from build123d import *

# Parameters (mm, degrees)
EXTRUDE_2_DEPTH     = 60
CUT_EXTRUDE_2_DEPTH = 189.939286944
SKETCH_7_R          = 25
CUT_EXTRUDE_4_DEPTH = 20
SKETCH_8_R          = 25
CUT_EXTRUDE_5_DEPTH = 20
SKETCH_9_W          = 30
SKETCH_9_H          = 70
CUT_EXTRUDE_6_DEPTH = 20
SKETCH_10_W         = 30
SKETCH_10_H         = 70
CUT_EXTRUDE_7_DEPTH = 20
FILLET_1_R          = 3
FILLET_2_R          = 3
FILLET_3_R          = 3
FILLET_4_R          = 3


with BuildPart() as part:
    # 草图1 → 凸台-拉伸2 (new body)
    with BuildSketch(Plane.XY):
        Polygon((-161.784091828, 76.967277349), (-161.784091828, 16.967277349), (-127.826106531, -63.032722651), (-27.826106531, -63.032722651), (6.131878766, 16.967277349), (6.131878766, 76.967277349), align=None)
    extrude(amount=EXTRUDE_2_DEPTH)

    # 草图5 → 切除-拉伸2 (cut, through all)
    with BuildSketch(Plane.XY.offset(60)):
        Polygon((-141.784091828, 76.967277349), (-141.784091828, 16.967277349), (-112.836441026, -51.229114277), (-42.815772036, -51.229114277), (-13.868121234, 16.967277349), (-13.868121234, 76.967277349), align=None)
    extrude(amount=-CUT_EXTRUDE_2_DEPTH, mode=Mode.SUBTRACT)

    # 草图7 → 切除-拉伸4 (cut)
    with BuildSketch(Plane.ZY.offset(161.784091828)):
        with Locations(Location((30, 46.967277349, 0), (0, 0, 270))):
            Circle(SKETCH_7_R)
    extrude(amount=-CUT_EXTRUDE_4_DEPTH, mode=Mode.SUBTRACT)

    # 草图8 → 切除-拉伸5 (cut)
    with BuildSketch(Plane(origin=(0, -51.229114277, 0), x_dir=(1, 0, 0), z_dir=(0, 1, 0))):
        with Locations(Location((-77.815772036, -30, 0), (0, 0, 270))):
            Circle(SKETCH_8_R)
    extrude(amount=-CUT_EXTRUDE_5_DEPTH, mode=Mode.SUBTRACT)

    # 草图9 → 切除-拉伸6 (cut)
    with BuildSketch(Plane(origin=(-130.981763761, -55.598460099, 0), x_dir=(0, 0, 1), z_dir=(-0.9205048534524416, -0.3907311284892711, 0))):
        with Locations((30, 36.923711729)):
            Rectangle(SKETCH_9_W, SKETCH_9_H)
    extrude(amount=-CUT_EXTRUDE_6_DEPTH, mode=Mode.SUBTRACT)

    # 草图10 → 切除-拉伸7 (cut)
    with BuildSketch(Plane(origin=(-0.906899112, 0.384955834, 0), x_dir=(0, 0, -1), z_dir=(0.9205048534524416, -0.3907311284892711, 0))):
        with Locations((-29.473403637, -23.894453133)):
            Rectangle(SKETCH_10_W, SKETCH_10_H)
    extrude(amount=-CUT_EXTRUDE_7_DEPTH, mode=Mode.SUBTRACT)

    # 圆角1
    fillet_1_edges = [part.edges().sort_by_distance(p)[0] for p in [
        (-144.805099179, -23.032722651, 0),
    ]]
    fillet(fillet_1_edges, radius=FILLET_1_R)

    # 圆角2
    fillet_2_edges = [part.edges().sort_by_distance(p)[0] for p in [
        (-144.805099179, -23.032722651, 60),
    ]]
    fillet(fillet_2_edges, radius=FILLET_2_R)

    # 圆角3
    fillet_3_edges = [part.edges().sort_by_distance(p)[0] for p in [
        (-10.847113883, -23.032722651, 60),
    ]]
    fillet(fillet_3_edges, radius=FILLET_3_R)

    # 圆角4
    fillet_4_edges = [part.edges().sort_by_distance(p)[0] for p in [
        (-10.847113883, -23.032722651, 0),
    ]]
    fillet(fillet_4_edges, radius=FILLET_4_R)


solid = part.part
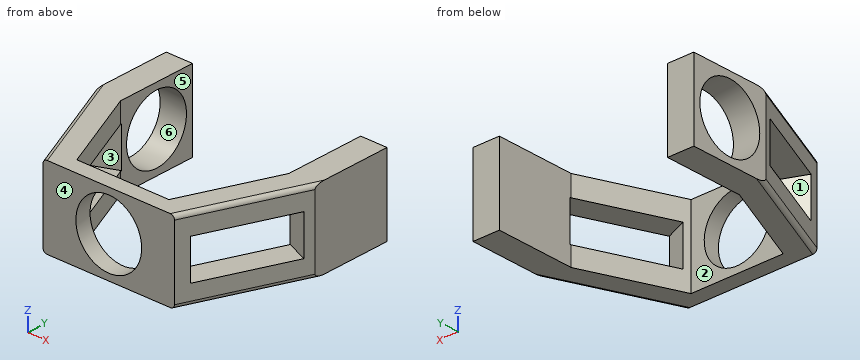
Work out the finished part from the listing and answer in its coordinate system (mm). Face numbers are marked on the shaded views. A direction names the side the tool comes from. Round coordinates to 2 decimals unless told otherwise and drop trailing zeros. Write each loop counter-clockwise with the first axis right and the second up, starting at its lowest first coordinate (ties: lowest second). Pieces come first, ordered by that corner, then holes. Notation, with made-up numbers: (40, 36) - (73, 36) arc R15 ccw to (73, 53) - close; hole circle Ø2 at (22.5, 22.25). An arc over 180 degrees is marked (long way). Answer in a Markdown table with one row per item. Add a question column.
1. A cutting plane is placed at B-B, the plane x = -94. Determine the outline of the cut face in (y, z).
2. The mould has two halves that part along Y. Classify the marked faces 4, 5 and 6: +Y half, -Y half, draft (parallel to the pull), parting line (faces both ways), or undercut.
3. For the marked faces 1, 2 and 3, determine the directions among +Z, -Z, +X, -X, +Y, -Y from which every point of the face is accessible in a straight line to the end or side of a thin tool.
4. A cutting plane is placed at A-A, the plane z = 30. Determine the outline of the cut face in (x, y), and give its area (3 significant figures).
5. Given pin 1 (5 mm diameter, centred on x = -40.5, z = 9.5, fed in from +Y); pin 2 (6 mm diameter, centred on y = 51.5, z = 9.5, fed in from -X); pin 3 (12 mm diameter, centred on x = -76.5, z = 11.5, fed in from -Y); pin 4 (4 mm diameter, centred on x = -25, z = 35, fed in from -Y), each flat-ended and moving along its own axis, determine where each tip first touches the part or whether it passes through.
6. A cutting plane is placed at C-C, the plane y = 42. Determine the outline of the cut face in (x, z).
7. A cutting plane is placed at D-D, the plane z = 48. Determine the outline of the cut face in (x, y).
8. Find the intervals of material crossed by line 1 along X through (y, z) = (23.5, 10.5); line 2 along X through (y, z) = (62.5, 24.5); line 3 along Y through (x, z) = (-47, 33), in increasing order. Write a range as from..to.
Worked out:
| question | item | result |
|---|---|---|
| 1 | outline | (-63.03, 0) - (-51.23, 0) - (-51.23, 10.95) - (-63.03, 10.95) - close; (-63.03, 49.05) - (-51.23, 49.05) - (-51.23, 60) - (-63.03, 60) - close |
| 2 | face 4 | -Y half |
| 2 | face 5 | draft |
| 2 | face 6 | undercut |
| 3 | face 1 | -X, +Y |
| 3 | face 2 | +Z, -Z, +Y |
| 3 | face 3 | -Y |
| 4 | outline | (-161.78, 16.97) - (-159.08, 10.61) - (-141.78, 17.95) - (-141.78, 21.97) - (-161.78, 21.97) - close; (-161.78, 71.97) - (-141.78, 71.97) - (-141.78, 76.97) - (-161.78, 76.97) - close; (-131.73, -53.83) - (-127.83, -63.03) - (-102.82, -63.03) - (-102.82, -51.23) - (-112.84, -51.23) - (-114.79, -46.63) - close; (-52.82, -63.03) - (-27.83, -63.03) - (-23.92, -53.83) - (-40.87, -46.63) - (-42.82, -51.23) - (-52.82, -51.23) - close; (-13.87, 17.95) - (3.43, 10.61) - (6.13, 16.97) - (6.13, 76.97) - (-13.87, 76.97) - close |
| 4 | area | 2,200 mm^2 |
| 5 | pin 1 | y = -39.88 |
| 5 | pin 2 | x = -13.87 |
| 5 | pin 3 | through |
| 5 | pin 4 | y = -61.09 |
| 6 | outline | (-161.78, 0) - (-141.78, 0) - (-141.78, 5.5) - (-161.78, 5.5) - close; (-161.78, 54.5) - (-141.78, 54.5) - (-141.78, 60) - (-161.78, 60) - close; (-13.87, 0) - (6.13, 0) - (6.13, 60) - (-13.87, 60) - close |
| 7 | outline | (-161.78, 16.97) - (-127.83, -63.03) - (-95.17, -63.03) - (-95.17, -51.23) - (-112.84, -51.23) - (-141.78, 16.97) - (-141.78, 29.62) - (-161.78, 29.62) - close; (-161.78, 64.32) - (-141.78, 64.32) - (-141.78, 76.97) - (-161.78, 76.97) - close; (-60.47, -63.03) - (-27.83, -63.03) - (6.13, 16.97) - (6.13, 76.97) - (-13.87, 76.97) - (-13.87, 16.97) - (-42.82, -51.23) - (-60.47, -51.23) - close |
| 8 | line 1 | -161.78..-141.78, -13.87..6.13 |
| 8 | line 2 | -13.87..6.13 |
| 8 | line 3 | -63.03..-51.23 |
